```python
from build123d import *

# Parameters (mm, degrees)
ESQUISSE13_R        = 1.5
ESQUISSE13_W        = 3
ESQUISSE13_H        = 6
ESQUISSE13_W_2      = 10
ESQUISSE13_H_2      = 3
ESQUISSE13_W_3      = 23
ESQUISSE13_H_3      = 11.8
BOSS_EXTRU_13_DEPTH = 3


with BuildPart() as part:
    # Esquisse13 → Boss.-Extru.13 (new body)
    with BuildSketch(Plane.XY):
        with BuildLine():
            Line((157.12523298, -14.425795559), (103.12523298, -14.425795559))
            ThreePointArc((103.12523298, -14.425795559), (101.003912637, -13.547115902), (100.12523298, -11.425795559))
            Line((100.12523298, -11.425795559), (100.12523298, 27.781080254))
            ThreePointArc((100.12523298, 27.781080254), (100.827637897, 29.710084358), (102.605937537, 30.735793817))
            Line((102.605937537, 30.735793817), (150.512449504, 39.155436821))
            ThreePointArc((150.512449504, 39.155436821), (152.911964034, 38.833240365), (154.686087677, 37.185828505))
            Line((154.686087677, 37.185828505), (159.736166166, 28.261732306))
            ThreePointArc((159.736166166, 28.261732306), (160.02633618, 27.548162294), (160.12523298, 26.784224979))
            Line((160.12523298, 26.784224979), (160.12523298, -11.425795559))
            ThreePointArc((160.12523298, -11.425795559), (159.246553324, -13.547115902), (157.12523298, -14.425795559))
        make_face()
        with Locations((151.204843429, 35.215818737)):
            Circle(ESQUISSE13_R, mode=Mode.SUBTRACT)
        with Locations((130.12523298, -9.925795559)):
            Circle(ESQUISSE13_R, mode=Mode.SUBTRACT)
        with Locations((120.62523298, 8.974204441)):
            Circle(ESQUISSE13_R, mode=Mode.SUBTRACT)
        with Locations((120.62523298, 27.974204441)):
            Circle(ESQUISSE13_R, mode=Mode.SUBTRACT)
        with Locations((155.62523298, -1.925795559)):
            Circle(ESQUISSE13_R, mode=Mode.SUBTRACT)
        with Locations((104.62523298, -1.925795559)):
            Circle(ESQUISSE13_R, mode=Mode.SUBTRACT)
        with Locations((104.62523298, -8.425795559)):
            Rectangle(ESQUISSE13_W, ESQUISSE13_H, mode=Mode.SUBTRACT)
        with Locations((112.62523298, -9.925795559)):
            Rectangle(ESQUISSE13_W_2, ESQUISSE13_H_2, mode=Mode.SUBTRACT)
        with Locations((155.62523298, -8.425795559)):
            Rectangle(ESQUISSE13_W, ESQUISSE13_H, mode=Mode.SUBTRACT)
        with Locations((147.62523298, -9.925795559)):
            Rectangle(ESQUISSE13_W_2, ESQUISSE13_H_2, mode=Mode.SUBTRACT)
        with Locations((104.62523298, 4.574204441)):
            Rectangle(ESQUISSE13_W, ESQUISSE13_H, mode=Mode.SUBTRACT)
        with Locations((155.62523298, 4.574204441)):
            Rectangle(ESQUISSE13_W, ESQUISSE13_H, mode=Mode.SUBTRACT)
        with Locations((120.62523298, 18.474204441)):
            Rectangle(ESQUISSE13_W_3, ESQUISSE13_H_3, mode=Mode.SUBTRACT)
    extrude(amount=BOSS_EXTRU_13_DEPTH)


solid = part.part
```
Verification items for the finished model (mm, model axes). A direction names the side the tool comes from. Round coordinates to 2 decimals unless told otherwise and drop trailing zeros. Write each loop counter-clockwise with the first axis right and the second up, starting at its lowest first coordinate (ties: lowest second). Pieces come first, ordered by that corner, then holes.
1. Scan lines: L1, parallel to X at y = 7, z = 2.55; L2, parallel to X at y = 18, z = 2.15; L3, parallel to Y at x = 121, z = 0.7. Record each from-to range of solid material in increasing order.
2. Access from +Z, -Z, +X, -X, +Y, -Y to the whole of each face (thin tool, end or side, straight path). Record for faces 4 (the flat face through (131, -14.426, 1)), 5 (the flat face through (156, 7.574, 1)).
3. Section check A-A on y = 15. Enter the section's corners in (x, z).
4. Section check B-B on x = 112. Enter the section's corners in (y, z), plus the area to 3 significant figures.
5. Section check C-C on x = 144. Enter the section's corners in (y, z).
6. Gauge pin test, flat ends, axial feed: P1, Ø2.5, axis at x = 120.63, y = 27.97, coming from the -Z side; P2, Ø1, axis at x = 113, z = 1, coming from the +Y side; P3, Ø0.9, axis at x = 110, z = 1.5, coming from the +Y side. Record the tip position at first contact, or that the pin passes through.
7. Section check D-D on z = 2.45. State how many separate pieces and enclosed holes the cut face has, plus the area to 3 significant figures.
8. Draft check along Y on faces 1 (the flat face through (157.125, -8, 1)), 2 (the flat face through (157.176, 32.786, 1.479)), 3 (the flat face through (137, 13, 3)). Enter one of: +Y half, -Y half, draft (parallel to the pull), parting line (faces both ways), or undercut.
Answer:
1. L1: x = 100.13 to 103.13, 106.13 to 154.13, 157.13 to 160.13
1. L2: x = 100.13 to 109.13, 132.13 to 160.13
1. L3: y = -14.43 to 7.52, 10.43 to 12.57, 24.37 to 26.52, 29.43 to 33.97
2. face 4: +Z, -Z, +X, -X, -Y
2. face 5: +Z, -Z
3. outline: (100.13, 0) - (109.13, 0) - (109.13, 3) - (100.13, 3) - close; (132.13, 0) - (160.13, 0) - (160.13, 3) - (132.13, 3) - close
4. outline: (-14.43, 0) - (-11.43, 0) - (-11.43, 3) - (-14.43, 3) - close; (-8.43, 0) - (12.57, 0) - (12.57, 3) - (-8.43, 3) - close; (24.37, 0) - (32.39, 0) - (32.39, 3) - (24.37, 3) - close
4. area: 96.0 mm2
5. outline: (-14.43, 0) - (-11.43, 0) - (-11.43, 3) - (-14.43, 3) - close; (-8.43, 0) - (38.01, 0) - (38.01, 3) - (-8.43, 3) - close
6. P1: passes through
6. P2: stops at y = 32.65
6. P3: stops at y = 32.11
7. separate pieces: 1
7. enclosed holes: 13
7. area: 2,500 mm2
8. face 1: undercut
8. face 2: +Y half
8. face 3: draft
